Could you check a few things on this model? Use its own coordinates, in mm. A direction names the side the tool comes from. Coordinates: 2 decimals unless noted, no trailing zeros. Write each loop counter-clockwise with the first axis right and the second up, starting at its lowest first coordinate (ties: lowest second). Pieces come first, ordered by that corner, then holes.
Item 1: For P1, Ø6.5, axis at x = 8, y = -16, coming from the +Z side; P2, Ø5.5, axis at x = 5.5, z = -9.5, coming from the -Y side, each with a flat end and sliding along its axis, tell me the tip position at first contact or that it passes through.
Item 2: Which directions (+Z, -Z, +X, -X, +Y, -Y) give clear straight access to the entire face, cutting with the end or side of a thin tool? Please do faces 5 (the flat face through (10, -13, -29)), 6 (the flat face through (9.9, -7, -6.7)), 7 (the cylindrical face through (8.5, -6.49, -5.23)).
Item 3: I want a section at B-B on z = -10. Please give me the cut outline in (x, y), then the cut area to 3 significant figures.
Item 4: Thinking about a two-plate mould opening in Z: for faces 1 (the flat face through (10, -13, -35)), 2 (the flat face through (0, -9, -30)), 3 (the cylindrical face through (10.1, -3.8, -6.9)), 4 (the flat face through (11, -14, -31)), which applies, +Z half, -Z half, draft (parallel to the pull), parting line (faces both ways), or undercut?
Item 5: I want a section at A-A on x = 10. State how many separate pieces and enclosed holes the cut face has, then the cut area to 3 significant figures.
Item 6: I want a section at D-D on z = -18.5. Please give me the cut outline in (x, y), then the cut area to 3 significant figures.
Item 7: I want a section at C-C on y = -9. Please give me the cut outline in (x, z), then the cut area to 4 significant figures.
Item 8: If I drill on probe 1 along Y at (x, z) = (10, -32); probe 2 along X at (y, z) = (-2, -10); probe 3 along Z at (x, y) = (1.75, -10.75), over which ranges is the centre line in solid material (lowest first)?
from build123d import *

# Parameters (mm, degrees)
SKETCH_1_W          = 20
SKETCH_1_H          = 28
EXTRUDE_1_DEPTH     = 5
SKETCH_1_3_W        = 20
SKETCH_1_3_H        = 7
EXTRUDE_2_DEPTH     = 27
SKETCH_2_R          = 5
EXTRUDE_3_DEPTH     = 2
SKETCH_5_R          = 2.75
CUT_EXTRUDE_2_DEPTH = 49.518037883
FILLET_1_R          = 1
SKETCH_6_R          = 3.1
CUT_EXTRUDE_3_DEPTH = 46
CUT_EXTRUDE_4_DEPTH = 3
CHAMFER_1_SIZE      = 5
CHAMFER_2_SIZE      = 0.5


with BuildPart() as part:
    # 草图1 → 凸台-拉伸1 (new body)
    with BuildSketch(Plane(origin=(0, 0, 0), x_dir=(1, 0, 0), z_dir=(0, 1, 0))):
        with Locations((10, 14)):
            Rectangle(SKETCH_1_W, SKETCH_1_H)
    extrude(amount=-EXTRUDE_1_DEPTH)

    # 草图1<3> → 凸台-拉伸2 (add)
    with BuildSketch(Plane(origin=(0, 0, 0), x_dir=(1, 0, 0), z_dir=(0, 1, 0))):
        with Locations((10, 31.5)):
            Rectangle(SKETCH_1_3_W, SKETCH_1_3_H)
    extrude(amount=-EXTRUDE_2_DEPTH)

    # 草图2 → 凸台-拉伸3 (add)
    with BuildSketch(Plane.XZ.offset(5)):
        with Locations(Location((10, -10, 0), (0, 0, 90))):
            Circle(SKETCH_2_R)
    extrude(amount=EXTRUDE_3_DEPTH)

    # 草图5 → 切除-拉伸2 (cut, through all)
    with BuildSketch(Plane(origin=(0, 0, -35), x_dir=(-1, 0, 0), z_dir=(0, 0, -1))):
        with Locations((-10, -17)):
            Circle(SKETCH_5_R)
    extrude(amount=-CUT_EXTRUDE_2_DEPTH, mode=Mode.SUBTRACT)

    # 圆角1
    fillet_1_edges = [part.edges().sort_by_distance(p)[0] for p in [
        (10, -5, -15),
    ]]
    fillet(fillet_1_edges, radius=FILLET_1_R)

    # 草图6 → 切除-拉伸3 (cut, through all)
    with BuildSketch(Plane.XZ.offset(7)):
        with Locations(Location((10, -10, 0), (0, 0, 270))):
            Circle(SKETCH_6_R)
    extrude(amount=-CUT_EXTRUDE_3_DEPTH, mode=Mode.SUBTRACT)

    # 草图7 → 切除-拉伸4 (cut)
    with BuildSketch(Plane.XY.offset(-28)):
        Polygon((14.618802154, -17), (12.309401077, -13), (7.690598923, -13), (5.381197846, -17), (7.690598923, -21), (12.309401077, -21), align=None)
    extrude(amount=-CUT_EXTRUDE_4_DEPTH, mode=Mode.SUBTRACT)

    # 倒角1
    chamfer_1_edges = [part.edges().sort_by_distance(p)[0] for p in [
        (0, -2.5, 0),
        (20, -2.5, 0),
    ]]
    chamfer(chamfer_1_edges, length=CHAMFER_1_SIZE)

    # 倒角2
    chamfer_2_edges = [part.edges().sort_by_distance(p)[0] for p in [
        (20, -16, -28),
        (0, -16, -28),
        (10, 0, -35),
        (10, -5, -28),
        (0, -13.5, -35),
        (20, -13.5, -35),
        (10, -27, -35),
        (12.75, -17, -35),
        (10, 0, -6.9),
        (10, 0, 0),
        (10, -5, 0),
        (20, 0, -20),
        (0, 0, -20),
        (2.5, 0, -2.5),
        (17.5, 0, -2.5),
        (20, -5, -16.5),
        (0, -5, -16.5),
        (2.5, -5, -2.5),
        (17.5, -5, -2.5),
    ]]
    chamfer(chamfer_2_edges, length=CHAMFER_2_SIZE)


solid = part.part
Response values:
1. P1: stops at z = -28
1. P2: stops at y = -7
2. face 5: +Z
2. face 6: +Z, +X, -X, -Y
2. face 7: -Y
3. outline: (0, -4.5) - (0.5, -5) - (4, -5) arc R1 cw to (5, -6) - (5, -7) - (6.9, -7) - (6.9, -0.5) - (6.4, 0) - (0.5, 0) - (0, -0.5) - close; (13.1, -7) - (15, -7) - (15, -6) arc R1 cw to (16, -5) - (19.5, -5) - (20, -4.5) - (20, -0.5) - (19.5, 0) - (13.6, 0) - (13.1, -0.5) - close
3. area: 76.3 mm2
4. face 1: -Z half
4. face 2: draft
4. face 3: undercut
4. face 4: +Z half
5. separate pieces: 3
5. enclosed holes: 0
5. area: 259 mm2
6. outline: (0, -4.5) - (0.5, -5) - (19.5, -5) - (20, -4.5) - (20, -0.5) - (19.5, 0) - (0.5, 0) - (0, -0.5) - close
6. area: 99.5 mm2
7. outline: (0, -34.5) - (0.5, -35) - (19.5, -35) - (20, -34.5) - (20, -28.5) - (19.5, -28) - (0.5, -28) - (0, -28.5) - close
7. area: 139.5 mm2
8. probe 1: y = -27 to -19.75, -14.25 to 0
8. probe 2: x = 0 to 6.9, 13.1 to 20
8. probe 3: z = -35 to -28
